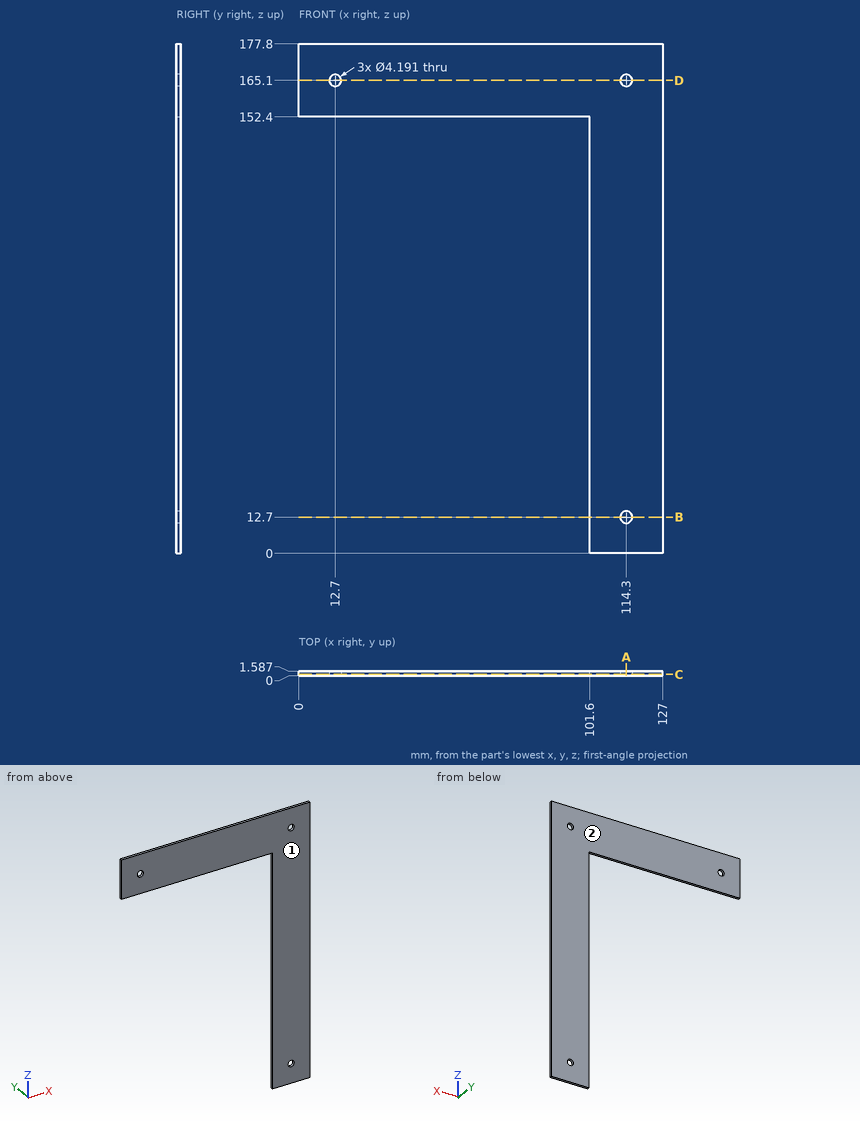
The figure shows three views and two pictorial views of one solid part (mm, origin at its lowest corner). Answer the questions. Give positions to 0.01 mm unless a question says otherwise; leave off trailing zeros. Write each loop counter-clockwise with the first axis right and the second up, starting at its lowest first coordinate (ties: lowest second). Pieces come first, ordered by that corner, then holes. Notation, with made-up numbers: (74.5, 8.25) - (114.5, 8.25) arc R7 cw to (114.5, 18.25) - close; hole circle Ø4 at (78.25, 27.25). An arc over 180 degrees is marked (long way). Use CSV: the item, a comma, the result in double quotes. Start each with the question number.
Item 1: The mould has two halves that part along Y. Classify the marked faces 1 and 2: pulls with the +Y half, pulls with the -Y half, needs draft (parallel to the pull), parting line crosses it, or undercut.
Item 2: The part is cut by section C-C, the plane y = 0.55. Give the vertices of the cut face in (x, z) (1 decimal).
Item 3: A flat-ended cylindrical pin translates along its axis: P1, Ø5, axis at x = 114.3, z = 165.1, coming from the +Y side. Find the tip coordinate at first contact, or state that the pin passes through.
Item 4: The part is cut by section D-D, the plane z = 165.1. Give the vertices of the cut face in (x, y) (1 decimal).
Item 5: The part is cut by section B-B, the plane z = 12.7. Give the vertices of the cut face in (x, y) (1 decimal).
Item 6: Consider line 1 (Z direction, x = 114.3, y = 0.45) (1 decimal); line 2 (Z direction, x = 25, y = 0.15); line 3 (X direction, y = 1, z = 12.7) (1 decimal). Determine where each line is inside the solid, lowest interval first.
Item 7: The part is cut by section A-A, the plane x = 114.3. Give the vertices of the cut face in (y, z) (1 decimal), and give its area (3 significant figures).
Taken from the geometry:
1,face 1,"pulls with the -Y half"
1,face 2,"pulls with the +Y half"
2,outline,"(0, 152.4) - (101.6, 152.4) - (101.6, 0) - (127, 0) - (127, 177.8) - (0, 177.8) - close; hole circle Ø4.2 at (12.7, 165.1); hole circle Ø4.2 at (114.3, 12.7); hole circle Ø4.2 at (114.3, 165.1)"
3,P1,"y = 1.59"
4,outline,"(0, 0) - (10.6, 0) - (10.6, 1.6) - (0, 1.6) - close; (14.8, 0) - (112.2, 0) - (112.2, 1.6) - (14.8, 1.6) - close; (116.4, 0) - (127, 0) - (127, 1.6) - (116.4, 1.6) - close"
5,outline,"(101.6, 0) - (112.2, 0) - (112.2, 1.6) - (101.6, 1.6) - close; (116.4, 0) - (127, 0) - (127, 1.6) - (116.4, 1.6) - close"
6,line 1,"0 to 10.6, 14.8 to 163, 167.2 to 177.8"
6,line 2,"152.4 to 177.8"
6,line 3,"101.6 to 112.2, 116.4 to 127"
7,outline,"(0, 0) - (1.6, 0) - (1.6, 10.6) - (0, 10.6) - close; (0, 14.8) - (1.6, 14.8) - (1.6, 163) - (0, 163) - close; (0, 167.2) - (1.6, 167.2) - (1.6, 177.8) - (0, 177.8) - close"
7,area,"269 mm2"
